Part print with two shaded views. Sizes in mm from the minimum x, y, z corner. A direction names the side the tool comes from. Give positions to 0.01 mm unless a question says otherwise; leave off trailing zeros. Write each loop counter-clockwise with the first axis right and the second up, starting at its lowest first coordinate (ties: lowest second). Pieces come first, ordered by that corner, then holes. Notation, with made-up numbers: (17.25, 50) -> (42.25, 50) arc R15 ccw to (42.25, 56) -> close; hole circle Ø8 at (-8.5, 82). An arc over 180 degrees is marked (long way). Use one line per item in the form item = value. Start each with the question number.
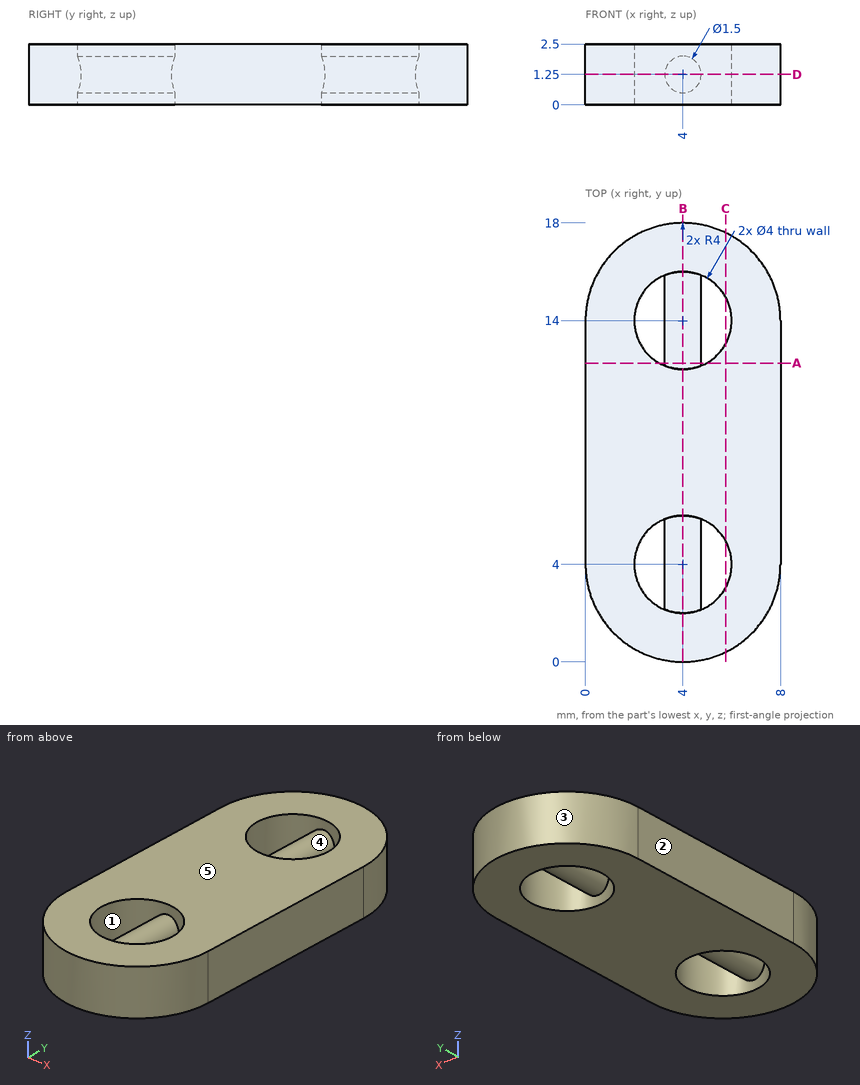
1) Cut at D-D (z = 1.25). Give the cut face in (x, y).
2) Cut at A-A (y = 12.25). Give the cut face in (x, z), and give its area (3 significant figures).
3) Cut at C-C (x = 5.75). Give the cut face in (y, z).
4) Wall check: line 1 along Y through (x, z) = (2.5, 0.3); line 2 along Y through (x, z) = (3.5, 0.45); line 3 along X through (y, z) = (13.75, 0.95). Give the ranges that are in metal, low to high. Write a range as from..to.
5) Cut at B-B (x = 4). Give the cut face in (y, z), and give its area (3 significant figures).
6) Two-plate mould, pull along Y, no slides. Class the marked faces 1, 2 and 3: released by +Y, released by -Y, zero draft, split by the parting line, or undercut.
7) 3-axis set-ups, long thin cutter, end or side, ignore diameter. For the marked faces 4 and 5: which of +Z, -Z, +X, -X, +Y, -Y reach the whole face in a straight line?
Final values:
q1.outline = (0, 4) arc R4 ccw to (8, 4) -> (8, 14) arc R4 ccw to (0, 14) -> close; hole (3.25, 2.15) -> (3.25, 5.85) arc R2 ccw to start; hole (3.25, 12.15) -> (3.25, 15.85) arc R2 ccw to start; hole (4.75, 2.15) arc R2 ccw to (4.75, 5.85) -> close; hole (4.75, 12.15) arc R2 ccw to (4.75, 15.85) -> close
q2.outline = (0, 0) -> (3.03, 0) -> (3.03, 2.5) -> (0, 2.5) -> close; circle Ø1.5 at (4, 1.25); (4.97, 0) -> (8, 0) -> (8, 2.5) -> (4.97, 2.5) -> close
q2.area = 16.9 mm^2
q3.outline = (0.4, 0) -> (3.03, 0) -> (3.03, 2.5) -> (0.4, 2.5) -> close; (4.97, 0) -> (13.03, 0) -> (13.03, 2.5) -> (4.97, 2.5) -> close; (14.97, 0) -> (17.6, 0) -> (17.6, 2.5) -> (14.97, 2.5) -> close
q4.line_1 = 0.29..2.68, 5.32..12.68, 15.32..17.71
q4.line_2 = 0.03..2.06, 5.94..12.06, 15.94..17.97
q4.line_3 = 0..2.02, 3.31..4.69, 5.98..8
q5.outline = (0, 0) -> (2, 0) -> (2, 0.5) -> (6, 0.5) -> (6, 0) -> (12, 0) -> (12, 0.5) -> (16, 0.5) -> (16, 0) -> (18, 0) -> (18, 2.5) -> (16, 2.5) -> (16, 2) -> (12, 2) -> (12, 2.5) -> (6, 2.5) -> (6, 2) -> (2, 2) -> (2, 2.5) -> (0, 2.5) -> close
q5.area = 37.0 mm^2
q6.face_1 = undercut
q6.face_2 = zero draft
q6.face_3 = released by +Y
q7.face_4 = none
q7.face_5 = +Z, +X, -X, +Y, -Y
